Can you work these out from the model? Positions are in its coordinate system, mm. A direction names the side the tool comes from. Coordinates: 2 decimals unless noted, no trailing zeros. Return JSON: item names as keys, results as strings. Group by question number.
1) If we mould it in two halves opening along Y, with no side actions, what happens to faces 1 (the face through (-2, 3.175, 3)), 2 (the face through (6, 4, 0)), 3 (the face through (6, 4, 3.81))? For each: pulls with the +Y half, pulls with the -Y half, needs draft (parallel to the pull), parting line crosses it, or undercut.
2) Which directions (+Z, -Z, +X, -X, +Y, -Y) give clear straight access to the entire face, cutting with the end or side of a thin tool? Please do faces 4 (the face through (5.386, 0.423, 7.713)), 5 (the face through (15, 3.175, 2)), 6 (the face through (7, 1, 10.16)).
3) Imagine slicing it at B-B (z = 2.54). Give the number of separate pieces and of enclosed holes in the cut face, and give its area (3 significant figures).
4) For pin 1 Ø3 at (x, z) = (15.5, 3) entering from +Y (3 decimals); pin 2 Ø2 at (y, z) = (8, 1.5) entering from -X; pin 3 Ø1 at (y, z) = (2, 8) entering from -X, each with a flat end and sliding along its axis, tell me the tip position at first contact or that it passes through.
5) If I drill on line 1 along X through (y, z) = (1.75, 2.5); line 2 along X through (y, z) = (0.5, 2.75); line 3 along Y through (x, z) = (6.5, 5.75), over which ranges is the centre line in solid material (lowest first)?
```python
from build123d import *

# Parameters (mm, degrees)
SKETCH1_R               = 0.635
BOSS_EXTRUDE1_DEPTH     = 5.08
SKETCH2_R               = 4.445
SKETCH2_R_2             = 0.635
BOSS_EXTRUDE2_DEPTH     = 5.08
SKETCH3_R               = 3.2385
CUT_EXTRUDE1_DEPTH      = 6.35
FILLET1_R               = 0.254
FILLET2_R               = 2.54
FILLET3_R               = 1.27
SKETCH5_R               = 0.381
CUT_EXTRUDE3_DEPTH      = 83.603101422
CUT_EXTRUDE4_DEPTH      = 83.603101422
CUT_EXTRUDE4_DEPTH_BACK = 83.603101422
SKETCH7_W               = 65.357576663
SKETCH7_H               = 10.612338137
FILLET4_R               = 1.27


with BuildPart() as part:
    # Sketch1 → Boss-Extrude1 (new body)
    with BuildSketch(Plane.XY):
        with BuildLine():
            Line((0, 0), (76.64958, 0))
            Line((76.64958, 0), (81.72958, 0))
            Line((81.72958, 0), (81.72958, 3.175))
            Line((81.72958, 3.175), (76.64958, 3.175))
            Line((76.64958, 3.175), (75.06208, 3.175))
            Line((75.06208, 3.175), (75.06208, 4.7625))
            ThreePointArc((75.06208, 4.7625), (70.29958, 9.525), (65.53708, 4.7625))
            Line((65.53708, 4.7625), (65.53708, 3.175))
            Line((65.53708, 3.175), (11.1125, 3.175))
            Line((11.1125, 3.175), (11.1125, 4.7625))
            ThreePointArc((11.1125, 4.7625), (6.35, 9.525), (1.5875, 4.7625))
            Line((1.5875, 4.7625), (1.5875, 3.175))
            Line((1.5875, 3.175), (0, 3.175))
            Line((0, 3.175), (-5.08, 3.175))
            Line((-5.08, 3.175), (-5.08, 0))
            Line((-5.08, 0), (0, 0))
        make_face()
        with Locations((6.35, 4.7625)):
            Circle(SKETCH1_R, mode=Mode.SUBTRACT)
        with Locations((70.29958, 4.7625)):
            Circle(SKETCH1_R, mode=Mode.SUBTRACT)
    extrude(amount=BOSS_EXTRUDE1_DEPTH)

    # Sketch2 → Boss-Extrude2 (add)
    # profile 1 of 2: a face of its own
    with BuildSketch(Plane.XY.offset(5.08)):
        with Locations((6.35, 4.7625)):
            Circle(SKETCH2_R)
        with Locations((6.35, 4.7625)):
            Circle(SKETCH2_R_2, mode=Mode.SUBTRACT)
    # profile 2 of 2: a face of its own
    with BuildSketch(Plane.XY.offset(5.08)):
        with Locations((70.29958, 4.7625)):
            Circle(SKETCH2_R)
        with Locations((70.29958, 4.7625)):
            Circle(SKETCH2_R_2, mode=Mode.SUBTRACT)
    extrude(amount=BOSS_EXTRUDE2_DEPTH)

    # Sketch3 → Cut-Extrude1 (cut)
    with BuildSketch(Plane.XY.offset(10.16)):
        with Locations((6.35, 4.7625)):
            Circle(SKETCH3_R)
        with Locations((70.29958, 4.7625)):
            Circle(SKETCH3_R)
    extrude(amount=-CUT_EXTRUDE1_DEPTH, mode=Mode.SUBTRACT)

    # Fillet1
    fillet1_edges = [part.edges().sort_by_distance(p)[0] for p in [
        (1.905, 4.7625, 5.08),
        (65.85458, 4.7625, 5.08),
    ]]
    fillet(fillet1_edges, radius=FILLET1_R)

    # Fillet2
    fillet2_edges = [part.edges().sort_by_distance(p)[0] for p in [
        (75.06208, 3.175, 2.54),
        (11.1125, 3.175, 2.54),
        (65.53708, 3.175, 2.54),
        (1.5875, 3.175, 2.54),
    ]]
    fillet(fillet2_edges, radius=FILLET2_R)

    # Fillet3
    fillet3_edges = [part.edges().sort_by_distance(p)[0] for p in [
        (-5.08, 3.175, 2.54),
        (81.72958, 3.175, 2.54),
    ]]
    fillet(fillet3_edges, radius=FILLET3_R)

    # Sketch5 → Cut-Extrude3 (cut, through all)
    with BuildSketch(Plane(origin=(0, 3.175, 0), x_dir=(1, 0, 0), z_dir=(0, 1, 0))):
        with Locations(Location((-2.413, -2.54, 0), (0, 0, 180))):
            Circle(SKETCH5_R)
        with Locations(Location((79.06258, -2.54, 0), (0, 0, 180))):
            Circle(SKETCH5_R)
        with Locations(Location((61.53658, -2.54, 0), (0, 0, 180))):
            Circle(SKETCH5_R)
        with Locations(Location((15.113, -2.54, 0), (0, 0, 180))):
            Circle(SKETCH5_R)
    extrude(amount=-CUT_EXTRUDE3_DEPTH, mode=Mode.SUBTRACT)

    # Sketch7 → Cut-Extrude4 (cut, two sides: drawn at the far end of the back side and taken through both)
    with BuildSketch(Plane(origin=(0, 3.175, 0), x_dir=(1, 0, 0), z_dir=(0, 1, 0)).offset(-CUT_EXTRUDE4_DEPTH_BACK)):
        with Locations((50.458788332, -5.306169069)):
            Rectangle(SKETCH7_W, SKETCH7_H)
    extrude(amount=CUT_EXTRUDE4_DEPTH + CUT_EXTRUDE4_DEPTH_BACK, mode=Mode.SUBTRACT)

    # Fillet4
    fillet4_edges = [part.edges().sort_by_distance(p)[0] for p in [
        (17.78, 3.175, 2.54),
    ]]
    fillet(fillet4_edges, radius=FILLET4_R)


solid = part.part
```
Calculated:
{
 "1": {"face 1": "pulls with the +Y half", "face 2": "needs draft", "face 3": "undercut"},
 "2": {"face 4": "+Z", "face 5": "+Z, -Z, +X, +Y", "face 6": "+Z, +X, -X, +Y, -Y"},
 "3": {"separate pieces": "3", "enclosed holes": "1", "area": "119 mm2"},
 "4": {"pin 1": "y = 3.175", "pin 2": "x = 2.15", "pin 3": "x = 2.52"},
 "5": {"line 1": "-5.08 to -2.79, -2.03 to 14.73, 15.49 to 17.78", "line 2": "-5.08 to -2.73, -2.1 to 14.8, 15.43 to 17.78", "line 3": "0.32 to 1.53, 8 to 9.2"}
}
